Source: CAD feature listing. Evaluate the final solid. Frame: model axes, mm. Give positions to 0.01 mm unless a question says otherwise; leave off trailing zeros. Loops run counter-clockwise (first coordinate to the right, second up) from the corner with the lowest first, then second, coordinate; pieces in that order, holes last. Notation, with made-up numbers: (4, 86) - (37, 86) arc R9 cw to (37, 94) - close; hole circle Ø1 at (65, -12.75). An arc over 180 degrees is marked (long way). Write each question's results on one line, items separated by ' | '. Start each with the question number.
(1) Cut plane C-C on z = 1392.5. Return the cut outline in (x, y).
(2) Contact query for a flat-ended pin moving along its axis: pin 1 (6 mm diameter, centred on x = -7.5, y = 5, fed in from -Z). Output: stop coordinate, or through.
(3) Material intervals for line 1 along X through (y, z) = (-10, 906.5); line 2 along Y through (x, z) = (-10.5, 362), sorted ascending. Write a range as [from, to].
(4) Cut plane A-A on y = 5. Return the cut outline in (x, z).
from build123d import *

# Parameters (mm, degrees)
F1_DEPTH = 1600


with BuildPart() as f1:
    # F0 (on Top) → F1 (new body)
    with BuildSketch(Plane.XY):
        with BuildLine():
            ThreePointArc((12.5, 10), (11.767767, 11.767767), (10, 12.5))
            Line((10, 12.5), (-10, 12.5))
            ThreePointArc((-10, 12.5), (-11.767767, 11.767767), (-12.5, 10))
            Line((-12.5, 10), (-12.5, -10))
            ThreePointArc((-12.5, -10), (-11.767767, -11.767767), (-10, -12.5))
            Line((-10, -12.5), (10, -12.5))
            ThreePointArc((10, -12.5), (11.767767, -11.767767), (12.5, -10))
            Line((12.5, -10), (12.5, 10))
        make_face()
        with BuildLine():
            ThreePointArc((11, -10), (10.707107, -10.707107), (10, -11))
            Line((10, -11), (-10, -11))
            ThreePointArc((-10, -11), (-10.707107, -10.707107), (-11, -10))
            Line((-11, -10), (-11, 10))
            ThreePointArc((-11, 10), (-10.707107, 10.707107), (-10, 11))
            Line((-10, 11), (11, 11))
            Line((11, 11), (11, -10))
        make_face(mode=Mode.SUBTRACT)
    extrude(amount=F1_DEPTH)


solid = f1.part
Ans:
1) outline: (-12.5, -10) arc R2.5 ccw to (-10, -12.5) - (10, -12.5) arc R2.5 ccw to (12.5, -10) - (12.5, 10) arc R2.5 ccw to (10, 12.5) - (-10, 12.5) arc R2.5 ccw to (-12.5, 10) - close; hole (-11, -10) arc R1 ccw to (-10, -11) - (10, -11) arc R1 ccw to (11, -10) - (11, 11) - (-10, 11) arc R1 ccw to (-11, 10) - close
2) pin 1: through
3) line 1: [-12.5, -11], [11, 12.5] | line 2: [-12.45, -10.87], [10.87, 12.45]
4) outline: (-12.5, 0) - (-11, 0) - (-11, 1600) - (-12.5, 1600) - close; (11, 0) - (12.5, 0) - (12.5, 1600) - (11, 1600) - close
